```python
from build123d import *

# Parameters (mm, degrees)
SKETCH1_R                      = 8
SKETCH1_R_2                    = 2.25
BOSS_EXTRUDE1_DEPTH            = 44
CUT_EXTRUDE4_DEPTH             = 4
CUT_EXTRUDE5_DEPTH             = 103.107700493
F_4_5_4_5_DIAMETER_HOLE1_D     = 4.5
F_4_5_4_5_DIAMETER_HOLE1_DEPTH = 10
F_4_5_4_5_DIAMETER_HOLE1_TIP   = 1.351936393
CHAMFER1_SIZE                  = 1
F_3_3_3_3_DIAMETER_HOLE1_D     = 3.3
CUT_EXTRUDE6_DEPTH             = 103.107700536
CUT_EXTRUDE6_DEPTH_BACK        = 103.107700536


with BuildPart() as part:
    # Sketch1 → Boss-Extrude1 (new body)
    with BuildSketch(Plane(origin=(0, 0, 0), x_dir=(1, 0, 0), z_dir=(0, 1, 0))):
        with BuildLine():
            Line((-13.5, 0), (13.5, 0))
            Line((13.5, 0), (15.976995957, 46.142328626))
            ThreePointArc((15.976995957, 46.142328626), (13.793369664, 55.108202842), (7.021555451, 61.376987134))
            Line((7.021555451, 61.376987134), (-30.261527843, 79.585616959))
            ThreePointArc((-30.261527843, 79.585616959), (-41.624453455, 77.76637977), (-43.75141009, 66.457013833))
            Line((-43.75141009, 66.457013833), (-13.5, 0))
        make_face()
        with Locations(Location((0, 47, 0), (0, 0, 270))):
            Circle(SKETCH1_R, mode=Mode.SUBTRACT)
        with Locations(Location((-34.65, 70.6, 0), (0, 0, 270))):
            Circle(SKETCH1_R_2, mode=Mode.SUBTRACT)
    extrude(amount=BOSS_EXTRUDE1_DEPTH)

    # Sketch2 → Cut-Extrude4 (cut)
    with BuildSketch(Plane.XZ):
        Polygon((0, -30.75), (15.150710485, -30.75), (16.545133066, -56.725781169), (-44.65, -86.612781563), (-44.65, -30.75), align=None)
    extrude(amount=-CUT_EXTRUDE4_DEPTH, mode=Mode.SUBTRACT)

    # Sketch4 → Cut-Extrude5 (cut, through all)
    with BuildSketch(Plane.XY):
        Polygon((-16, 0), (-44.65, 37), (-44.65, 0), align=None)
    extrude(amount=-CUT_EXTRUDE5_DEPTH, mode=Mode.SUBTRACT)

    # Ø4.5 (4.5) Diameter Hole1
    with Locations(Plane(origin=(0, 4, 0), x_dir=(-1, 0, 0), z_dir=(0, -1, 0))):
        with Locations((0, 35), (0, 59), (12, 47), (-12, 47)):
            Hole(F_4_5_4_5_DIAMETER_HOLE1_D / 2, depth=F_4_5_4_5_DIAMETER_HOLE1_DEPTH)
            with Locations((0, 0, -(F_4_5_4_5_DIAMETER_HOLE1_DEPTH + F_4_5_4_5_DIAMETER_HOLE1_TIP / 2))):  # 118° drill point
                Cone(0, F_4_5_4_5_DIAMETER_HOLE1_D / 2, F_4_5_4_5_DIAMETER_HOLE1_TIP, mode=Mode.SUBTRACT)

    # Chamfer1
    chamfer1_edges = [part.edges().sort_by_distance(p)[0] for p in [
        (9.75, 4, -47),
        (-14.25, 4, -47),
        (-2.25, 4, -59),
        (-2.25, 4, -35),
        (-34.65, 44, -72.85),
    ]]
    chamfer(chamfer1_edges, length=CHAMFER1_SIZE)

    # Ø3.3 (3.3) Diameter Hole1 (through all)
    with Locations(Plane.XY):
        with Locations((-10, 32), (10, 32), (10, 12), (-10, 12)):
            Hole(F_3_3_3_3_DIAMETER_HOLE1_D / 2)

    # Sketch13 → Cut-Extrude6 (cut, two sides: drawn at the far end of the back side and taken through both)
    with BuildSketch(Plane(origin=(0, 0, 0), x_dir=(0, 0, -1), z_dir=(1, 0, 0)).offset(-CUT_EXTRUDE6_DEPTH_BACK)):
        with BuildLine():
            Line((10, 35.5), (25, 35.5))
            ThreePointArc((25, 35.5), (28.5, 32), (25, 28.5))
            Line((25, 28.5), (10, 28.5))
            Line((10, 28.5), (10, 35.5))
        make_face()
        with BuildLine():
            Line((10, 15.5), (25, 15.5))
            ThreePointArc((25, 15.5), (28.5, 12), (25, 8.5))
            Line((25, 8.5), (10, 8.5))
            Line((10, 8.5), (10, 15.5))
        make_face()
    extrude(amount=CUT_EXTRUDE6_DEPTH + CUT_EXTRUDE6_DEPTH_BACK, mode=Mode.SUBTRACT)


solid = part.part
```
Part model, mm, in its own coordinate system. A direction names the side the tool comes from. Round coordinates to 2 decimals unless told otherwise and drop trailing zeros. Loops run counter-clockwise (first coordinate to the right, second up) from the corner with the lowest first, then second, coordinate; pieces in that order, holes last.
Item 1: Cut at B-B, the plane x = -34.65. Give the cut face in (y, z).
Item 2: 3-axis set-ups, long thin cutter, end or side, ignore diameter. For faces 1 (the face through (-32.42, 34.36, -70.89)), 2 (the face through (-6, 32.1, -28.5)), 3 (the face through (1.038, 9.563, -57.004)): which of +Z, -Z, +X, -X, +Y, -Y reach the whole face in a straight line?
Item 3: Drill centre lines: line 1 (Y direction, x = -4.5, z = -14); line 2 (Y direction, x = 10, z = -4); line 3 (Z direction, x = 0, y = 8.25). Where is each one in solid material? Low to high.
Item 4: Cut at D-D, the plane z = -53. Give the cut face in (x, y), then the cut area to 3 significant figures.
Item 5: Cut at A-A, the plane y = 32. State how many separate pieces and enclosed holes the cut face has, then the cut area to 3 significant figures.
Item 6: Drop flat-ended pins along their axis: P1, Ø3, axis at x = -1, z = -65.5, coming from the -Y side; P2, Ø12, axis at y = 39.5, z = -21.5, coming from the -X side; P3, Ø5, axis at x = -0.5, y = 4.5, coming from the -Z side. Give the stop position or say it passes through.
Item 7: Mould opens along Y. For faces 4 (the face through (14.72, 21.69, -22.75)), 5 (the face through (0.051, 15.117, -59.387)), 6 (the face through (-2, 32, -10)) say: +Y half, -Y half, draft (parallel to the pull), parting line (faces both ways), or undercut.
A:
1. outline: (24.09, -80.6) - (44, -80.6) - (44, -73.85) - (43, -72.85) - (24.09, -72.85) - close; (24.09, -68.35) - (43, -68.35) - (44, -67.35) - (44, -46.46) - (24.09, -46.46) - close
2. face 1: +Y, -Y
2. face 2: +X, -X
2. face 3: -Y
3. line 1: y = 0 to 8.5, 15.5 to 28.5, 35.5 to 44
3. line 2: y = 0 to 10.35, 13.65 to 30.35, 33.65 to 44
3. line 3: z = -64.81 to -61.25, -56.75 to -55, -39 to -37.25, -32.75 to 0
4. outline: (-37.63, 27.93) - (-19.1, 4) - (-5.29, 4) - (-5.29, 44) - (-37.63, 44) - close; (5.29, 4) - (14.83, 4) - (14.83, 44) - (5.29, 44) - close; hole circle Ø3.3 at (-10, 12); hole circle Ø3.3 at (-10, 32); hole circle Ø3.3 at (10, 12); hole circle Ø3.3 at (10, 32)
4. area: 1,420 mm2
5. separate pieces: 6
5. enclosed holes: 2
5. area: 1,910 mm2
6. P1: stops at y = 4
6. P2: stops at x = -26.02
6. P3: stops at z = -66.27
7. face 4: draft
7. face 5: -Y half
7. face 6: undercut
